Work out the finished part from the listing and answer in its coordinate system (mm). A direction names the side the tool comes from. Coordinates: 2 decimals unless noted, no trailing zeros. Write each loop counter-clockwise with the first axis right and the second up, starting at its lowest first coordinate (ties: lowest second). Pieces come first, ordered by that corner, then holes. Notation, with made-up numbers: M 83,32 L 131,32 A28 cw 131,62 Z; hole C 21,31.5 d4. An arc over 180 degrees is marked long. Answer as CSV lines item,"result". Start each with the question number.
(1) Find the intervals of material crossed by L1, parallel to Y at x = 4.9, z = 9.5, in increasing order. Write a range as [from, to].
(2) Flat-ended cylindrical pins translate along their axes: P1, Ø0.6, axis at x = 2, z = 10, coming from the +Y side; P2, Ø5, axis at x = 5.5, z = 1.5, coming from the -Y side; P3, Ø5.5, axis at x = 10, z = 11, coming from the -Y side; P4, Ø0.6, axis at y = 9.5, z = 2, coming from the +X side. Find the tip coordinate at first contact, or state that the pin passes through.
(3) A cutting plane is placed at D-D on y = 13.5. Give the vertices of the cut face in (x, z), then the cut area to 3 significant figures.
(4) A cutting plane is placed at A-A on y = 9.5. Give the vertices of the cut face in (x, z).
(5) A cutting plane is placed at C-C on z = 6. Give the vertices of the cut face in (x, y).
(6) The mould has two halves that part along Z. Classify faces 4 (the flat face through (12, 13, 12)), 5 (the flat face through (4, 0, 4)), 6 (the cylindrical face through (5.958, 9.444, 8.237)): released by +Z, released by -Z, zero draft, split by the parting line, or undercut.
(7) For faces 1 (the cylindrical face through (9.444, 5.958, 10.763)), 2 (the flat face through (4, 10, 1)), 3 (the flat face through (4, 1, 12)), determine the directions among +Z, -Z, +X, -X, +Y, -Y from which every point of the face is accessible in a straight line to the end or side of a thin tool.
Autodesk Fusion 360 part; units mm, degrees
sketch "Sketch1" plane through (0, 0, 0) normal (0, 0, 1) x (1, 0, 0)
  line L0 (0, 0) -> (15, 0)
  line L1 (15, 0) -> (15, 15)
  line L2 (15, 15) -> (0, 15)
  line L3 (0, 15) -> (0, 0)
  dimension "d5" = 15
  dimension "d6" = 15
extrude "Extrude1" add sketch "Sketch1" along normal blind 15
sketch "Sketch2" plane through (0, 0, 0) normal (0, -1, 0) x (1, 0, 0)
  line L0 (0, 0) -> (15, 0)
  line L1 (15, 0) -> (15, 15)
  line L2 (15, 15) -> (0, 15)
  line L3 (0, 15) -> (0, 0)
  line L4 (4, 4) -> (15, 4)
  line L5 (15, 4) -> (15, 15)
  line L6 (15, 15) -> (4, 15)
  line L7 (4, 15) -> (4, 4)
  point P0 (4, 4)
  dimension "d9" = 4
  dimension "d10" = 4
extrude "Extrude2" cut sketch "Sketch2" against normal blind 3 contours L1 L2 L4 L5 L6 L7
sketch "Sketch3" plane through (0, 0, 0) normal (-1, 0, 0) x (0, -1, 0)
  line L0 (-15, 0) -> (0, 0)
  line L1 (0, 0) -> (0, 15)
  line L2 (0, 15) -> (-15, 15)
  line L3 (-15, 15) -> (-15, 0)
  line L4 (-4, 4) -> (-15, 4)
  line L5 (-15, 4) -> (-15, 15)
  line L6 (-15, 15) -> (-4, 15)
  line L7 (-4, 15) -> (-4, 4)
  point P0 (-4, 4)
  dimension "d14" = 4
  dimension "d15" = 4
extrude "Extrude3" cut sketch "Sketch3" against normal blind 3 contours L2 L3 L4 L5 L6 L7
sketch "Sketch4" plane through (0, 0, 0) normal (0, 0, -1) x (1, 0, 0)
  line L0 (0, 0) -> (0, -15)
  line L1 (0, -15) -> (15, -15)
  line L2 (15, -15) -> (15, 0)
  line L3 (15, 0) -> (0, 0)
  line L4 (4, -4) -> (15, -4)
  line L5 (15, -4) -> (15, -15)
  line L6 (15, -15) -> (4, -15)
  line L7 (4, -15) -> (4, -4)
  point P0 (4, -4)
  dimension "d18" = 4
  dimension "d19" = 4
extrude "Extrude4" cut sketch "Sketch4" against normal blind 3 contours L1 L2 L4 L5 L6 L7
sketch "Sketch5" plane through (0, 3, 0) normal (0, -1, 0) x (1, 0, 0)
  line L0 (4, 15) -> (4, 4)
  line L1 (4, 4) -> (15, 4)
  line L2 (15, 4) -> (15, 15)
  line L3 (15, 15) -> (4, 15)
  point P0 (9.5, 9.5)
  dimension "d42" = 5.5
  dimension "d43" = 5.5
sketch "Sketch6" plane through (3, 0, 0) normal (-1, 0, 0) x (0, -1, 0)
  line L0 (-4, 15) -> (-15, 15)
  line L1 (-15, 15) -> (-15, 4)
  line L2 (-15, 4) -> (-4, 4)
  line L3 (-4, 4) -> (-4, 15)
  point P0 (-9.5, 9.5)
  dimension "d44" = 5.5
  dimension "d45" = 5.5
sketch "Sketch7" plane through (0, 0, 3) normal (0, 0, -1) x (1, 0, 0)
  line L0 (4, -15) -> (15, -15)
  line L1 (15, -15) -> (15, -4)
  line L2 (15, -4) -> (4, -4)
  line L3 (4, -4) -> (4, -15)
  point P0 (9.5, -9.5)
  dimension "d46" = 5.5
  dimension "d47" = 5.5
hole "Hole4" at (9.5, 3, 9.5) direction (0, 1, 0) diameter 2.529 end through all countersink diameter 3 countersink angle 90
hole "Hole5" at (3, 9.5, 9.5) direction (1, 0, 0) diameter 2.529 end through all countersink diameter 3 countersink angle 90
hole "Hole6" at (9.5, 9.5, 3) direction (0, 0, 1) diameter 2.529 end through all countersink diameter 3 countersink angle 90
fillet "Fillet3" radius 5 3 edges at (4, 1.5, 4) (1.5, 4, 4) (4, 4, 1.5)
chamfer "Chamfer2" distance 4 angle 45 3 edges at (15, 9, 15) (15, 15, 9) (9, 15, 15)
fillet "Fillet4" radius 4 3 edges at (1.5, 4, 15) (15, 1.5, 4) (4, 15, 1.5)
equation "length_rib = 15 mm"
equation "distance_corner = 4 mm"
equation "distance_remaining = length_rib - distance_corner"
equation "distance_hole = distance_remaining / 2"
equation "d5 = length_rib"
equation "d6 = length_rib"
equation "d7 = length_rib"
equation "d9 = distance_corner"
equation "d10 = distance_corner"
equation "plate_thickness = 3 mm"
equation "d14 = distance_corner"
equation "d15 = distance_corner"
equation "d18 = distance_corner"
equation "d19 = distance_corner"
equation "d42 = distance_remaining / 2"
equation "d43 = distance_remaining / 2"
equation "d44 = distance_remaining / 2"
equation "d45 = distance_remaining / 2"
equation "d46 = distance_remaining / 2"
equation "d47 = distance_remaining / 2"
Here are the results:
1,L1,"y = [3, 8.24], [10.76, 15]"
2,P1,"stops at y = 4"
2,P2,"stops at y = 0"
2,P3,"stops at y = 3"
2,P4,"stops at x = 4"
3,outline,"M 0,0 L 3.12,0 L 3.12,3 L 12.5,3 L 12.5,11 L 11,12.5 L 3,12.5 L 3,4 L 0,4 Z; hole C 9.5,9.5 d2.53"
3,area,"96.5 mm^2"
4,outline,"M 0,0 L 4,0 L 4,3 L 8,3 L 8.24,3.24 L 8.24,8.24 L 3.24,8.24 L 3,8 L 3,4 L 0,4 Z; M 3,11 L 3.24,10.76 L 8.24,10.76 L 8.24,15 L 3,15 Z; M 10.76,3.24 L 11,3 L 15,3 L 15,8.24 L 10.76,8.24 Z; M 10.76,10.76 L 15,10.76 L 15,11 L 11,15 L 10.76,15 Z"
5,outline,"M 0,0 L 5,0 L 5,3 L 15,3 L 15,11 L 11,15 L 3,15 L 3,5 L 0,5 Z; hole C 9.5,9.5 d2.53"
6,face 4,"released by +Z"
6,face 5,"zero draft"
6,face 6,"undercut"
7,face 1,"+Y, -Y"
7,face 2,"-Z, +X, +Y"
7,face 3,"+Z, +X, -Y"
